```python
from build123d import *

# Parameters (mm, degrees)
F1_DEPTH  = 16
F2_R      = 1.7
F3_DEPTH  = 25
F5_DEPTH  = 25
F2_W      = 14.61311616
F2_H      = 5
F2_W_2    = 5
F2_H_2    = 11.9260823121
F6_DEPTH  = 2.5
F7_W      = 5.4
F7_H      = 10.7
F8_DEPTH  = 25
F9_R      = 2.5
F10_SIZE  = 1
F2_R_2    = 2.7
F11_DEPTH = 25


with BuildPart() as f1:
    # F0 (on Top) → F1 (new body)
    with BuildSketch(Plane.XY):
        Polygon((5, 20), (0, 20), (0, 0), (-20, 0), (-20, -15), (33, -15), (33, 0), (5, 0), align=None)
    extrude(amount=F1_DEPTH)

    # F2 (on face) → F3 (cut)
    with BuildSketch(Plane.XZ.offset(15)):
        with Locations((17, 3)):
            Circle(F2_R)
        with Locations((-2, 3)):
            Circle(F2_R)
    extrude(amount=-F3_DEPTH, mode=Mode.SUBTRACT)

    # F4 (on face) → F5 (cut)
    with BuildSketch(Plane(origin=(0, 0, 0), x_dir=(1, 0, 0), z_dir=(0, 0, -1))):
        Polygon((19.75, 12.3516352639), (17, 12.3516352639), (14.25, 12.3516352639), (14.25, 9.9516352639), (17, 9.9516352639), (19.75, 9.9516352639), align=None)
        Polygon((0.75, 12.0808439121), (-2, 12.0808439121), (-4.75, 12.0808439121), (-4.75, 9.6808439121), (-2, 9.6808439121), (0.75, 9.6808439121), align=None)
    extrude(amount=-F5_DEPTH, mode=Mode.SUBTRACT)

    # F2 (on face) → F6 (cut)
    with BuildSketch(Plane.XZ.offset(15)):
        with Locations((7.30655808, 8.5)):
            Rectangle(F2_W, F2_H)
        with Locations((23.2, 7.5428758864)):
            Rectangle(F2_W_2, F2_H_2)
    extrude(amount=-F6_DEPTH, mode=Mode.SUBTRACT)

    # F7 (on face) → F8 (cut)
    with BuildSketch(Plane.YZ.offset(5)):
        with Locations((10, 10.65)):
            Rectangle(F7_W, F7_H)
    extrude(amount=-F8_DEPTH, mode=Mode.SUBTRACT)

    # F9
    f9_edges = [f1.edges().sort_by_distance(p)[0] for p in [
        (2.5, 7.3, 5.3),
        (2.5, 12.7, 5.3),
        (2.5, 20, 16),
        (-20, -7.5, 16),
        (33, -7.5, 16),
        (2.5, 12.7, 16),
        (2.5, 7.3, 16),
        (5, 0, 8),
    ]]
    fillet(f9_edges, radius=F9_R)

    # F10
    f10_edges = [f1.edges().sort_by_distance(p)[0] for p in [
        (7.306558, -12.5, 11),
        (23.2, -12.5, 13.505917),
        (33, -7.5, 0),
        (-20, -7.5, 0),
        (2.5, 20, 0),
    ]]
    chamfer(f10_edges, length=F10_SIZE)

    # F2 (on face) → F11 (cut)
    with BuildSketch(Plane.XZ.offset(15)):
        with Locations((-10, 8)):
            Circle(F2_R_2)
    extrude(amount=-F11_DEPTH, mode=Mode.SUBTRACT)


solid = f1.part
```
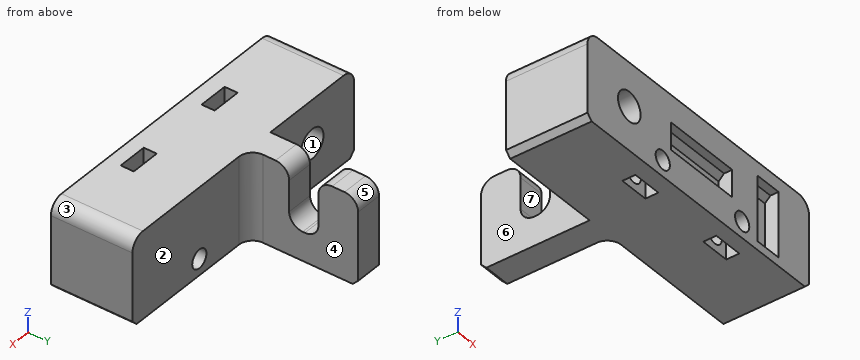
Model file for the job. Use its own axes, mm. Face numbers are marked on the shaded views. A direction names the side the tool comes from. Coordinates: 2 decimals unless noted, no trailing zeros. Loops run counter-clockwise (first coordinate to the right, second up) from the corner with the lowest first, then second, coordinate; pieces in that order, holes last. Notation, with made-up numbers: (11.25, 5.25) - (16.25, 5.25) arc R34 ccw to (16.25, 36.25) - close; hole circle Ø11 at (36, -7.75). An arc over 180 degrees is marked (long way). Write item = value, one per line. Start each with the question number.
Item 1: Drop flat-ended pins along their axis: pin 1 Ø2.5 at (x, z) = (24, 5.5) entering from -Y; pin 2 Ø3 at (x, z) = (13.5, 5) entering from +Y; pin 3 Ø6 at (y, z) = (12, 7) entering from -X. Give the stop position or say it passes through.
Item 2: Saw through at B-B, the plane z = 7. State how many separate pieces and enclosed holes the cut face has, then the cut area to 3 significant figures.
Item 3: Saw through at D-D, the plane y = -4. List the corners of the cut face in (x, z), then the cut area to 3 significant figures.
Item 4: Pull direction X, two halves, no side cores. Call the marked faces 1, 2 and 3: +X half, -X half, draft (parallel to the pull), parting line (faces both ways), or undercut.
Item 5: Saw through at C-C, the plane x = -10. List the corners of the cut face in (y, z).
Item 6: 3-axis set-ups, long thin cutter, end or side, ignore diameter. For the marked faces 4, 5, 6 and 7: which of +Z, -Z, +X, -X, +Y, -Y reach the whole face in a straight line?
Item 7: Wall check: probe 1 along X at (y, z) = (-13, 10.75); probe 2 along Y at (x, z) = (18, 10.5); probe 3 along Z at (x, y) = (-2, -14). Give the ranges that are in metal, low to high. Write a range as [from, to].
Item 8: Saw through at A-A, the plane x = -2. List the corners of the cut face in (y, z), then the cut area to 3 significant figures.
Answers:
q1.pin_1 = -12.5
q1.pin_2 = 0
q1.pin_3 = 0
q2.separate_pieces = 3
q2.enclosed_holes = 2
q2.area = 720 mm2
q3.outline = (-20, 1) - (-19, 0) - (32, 0) - (33, 1) - (33, 13.5) arc R2.5 ccw to (30.5, 16) - (-17.5, 16) arc R2.5 ccw to (-20, 13.5) - close; hole circle Ø5.4 at (-10, 8); hole circle Ø3.4 at (-2, 3); hole circle Ø3.4 at (17, 3)
q3.area = 803 mm2
q4.face_1 = undercut
q4.face_2 = draft
q4.face_3 = +X half
q5.outline = (-15, 0) - (0, 0) - (0, 5.3) - (-15, 5.3) - close; (-15, 10.7) - (0, 10.7) - (0, 16) - (-15, 16) - close
q6.face_4 = +Z, -Z, +X, +Y
q6.face_5 = +Z, +X, -X, +Y
q6.face_6 = +Z, -Z, -X, +Y
q6.face_7 = +Z, +X, -X
q7.probe_1 = [-20, 20.7], [25.7, 33]
q7.probe_2 = [-15, -12.35], [-9.95, 0]
q7.probe_3 = [0, 1.3], [4.7, 16]
q8.outline = (-15, 0) - (-12.08, 0) - (-12.08, 1.3) - (-15, 1.3) - close; (-15, 4.7) - (-12.08, 4.7) - (-12.08, 16) - (-15, 16) - close; (-9.68, 0) - (0, 0) - (0, 1.3) - (-9.68, 1.3) - close; (-9.68, 4.7) - (0, 4.7) - (0, 16) - (-9.68, 16) - close
q8.area = 159 mm2
